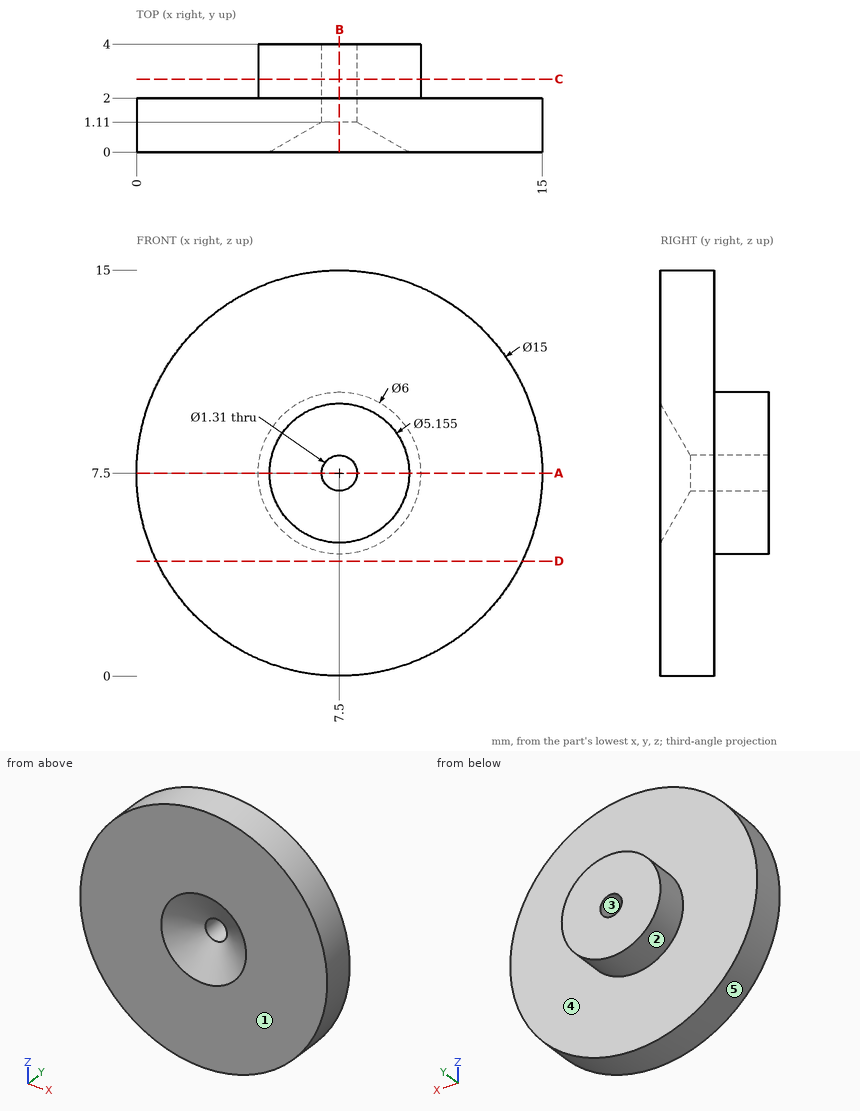
Geometry check sheet. Reference: drawing and pictorial views, mm from the part's lowest x, y, z. A direction names the side the tool comes from. Give positions to 0.01 mm unless a question says otherwise; leave off trailing zeros. Order: outer loops, then holes, each group sorted by start corner. A loop starts at its lowest first (then second) coordinate and runs counter-clockwise, first axis right, second up. Notation, with made-up numbers: M 8,-10.75 L 65,-10.75 A19 ccw 65,4.25 Z; hole C 54.25,67 d8. An arc over 180 degrees is marked long. Use one line per item in the form item = value. Start each with the question number.
Q1. Section check C-C (y = 2.7). Enter the section's corners in (x, z) (3 decimals), then the cut area to 3 significant figures.
Q2. Mould release check, pull along Z, two halves, no side actions. Record for the marked faces 1, 2 and 3: +Z half, -Z half, draft (parallel to the pull), parting line (faces both ways), or undercut.
Q3. Section check A-A (z = 7.5). Enter the section's corners in (x, y) (1 decimal).
Q4. Go/stop test with flat-tipped pins: pin 1 Ø2 at (x, z) = (7.5, 7.5) entering from -Y; pin 2 Ø1 at (x, y) = (12, 1) entering from -Z; pin 3 Ø1 at (x, z) = (12, 2.5) entering from +Y. Record where each tip stops, or that it passes through.
Q5. Section check D-D (z = 4.25). Enter the section's corners in (x, y).
Q6. Scan lines: line 1 along X through (y, z) = (2.3, 7.5) (3 decimals); line 2 along Z through (x, y) = (7.25, 2.25) (1 decimal); line 3 along Y through (x, z) = (6.75, 1.25). Record each from-to range of solid material in increasing order. Write a range as [from, to].
Q7. Access from +Z, -Z, +X, -X, +Y, -Y to the whole of each face (thin tool, end or side, straight path). Record for the marked faces 4 and 5.
Q8. Section check B-B (x = 7.5). Enter the section's corners in (y, z) (1 decimal), then the cut area to 3 significant figures.
Evaluation:
q1.outline = C 7.5,7.5 d6; hole C 7.5,7.5 d1.31
q1.area = 26.9 mm2
q2.face_1 = draft
q2.face_2 = parting line
q2.face_3 = undercut
q3.outline = M 0,0 L 4.9,0 L 6.8,1.1 L 6.8,4 L 4.5,4 L 4.5,2 L 0,2 Z; M 8.2,1.1 L 10.1,0 L 15,0 L 15,2 L 10.5,2 L 10.5,4 L 8.2,4 Z
q4.pin_1 = 0.91
q4.pin_2 = 1.16
q4.pin_3 = 2
q5.outline = M 0.74,0 L 14.26,0 L 14.26,2 L 0.74,2 Z
q6.line_1 = [4.5, 6.845], [8.155, 10.5]
q6.line_2 = [4.5, 6.9], [8.1, 10.5]
q6.line_3 = [0, 2]
q7.face_4 = +Y
q7.face_5 = +Y, -Y
q8.outline = M 0,0 L 2,0 L 2,4.5 L 4,4.5 L 4,6.8 L 1.1,6.8 L 0,4.9 Z; M 0,10.1 L 1.1,8.2 L 4,8.2 L 4,10.5 L 2,10.5 L 2,15 L 0,15 Z
q8.area = 34.6 mm2
